from build123d import *

# Parameters (mm, degrees)
SKETCH_1_R               = 6
EXTRUDE_1015_DEPTH       = 100
SKETCH_2_R               = 6.5
EXTRUDE_2_DEPTH          = 15
SKETCH_3_R               = 6
EXTRUDE_3_DEPTH          = 11
SKETCH_4_R               = 5.5
CUT_EXTRUDE_1_DEPTH      = 2
SKETCH_5_R               = 3.5
SKETCH_5_R_2             = 0.75
EXTRUDE_1402_DEPTH       = 2
SKETCH_6_W               = 1.5
SKETCH_6_H               = 0.8
EXTRUDE_1605_DEPTH       = 1
PATTERN_CIRCULAR_1_COUNT = 8


with BuildPart() as part:
    # Эскиз1 → Extrude 1015 (new body)
    with BuildSketch(Plane(origin=(0, 0, 0), x_dir=(1, 0, 0), z_dir=(0, 1, 0))):
        with Locations(Location((0, 0, 0), (0, 0, 270))):
            Circle(SKETCH_1_R)
    extrude(amount=EXTRUDE_1015_DEPTH)

    # Эскиз2 → Бобышка-Вытянуть2 (add)
    with BuildSketch(Plane(origin=(0, 100, 0), x_dir=(1, 0, 0), z_dir=(0, 1, 0))):
        with Locations(Location((0, 0, 0), (0, 0, 270))):
            Circle(SKETCH_2_R)
    extrude(amount=EXTRUDE_2_DEPTH)

    # Эскиз3 → Бобышка-Вытянуть3 (add)
    with BuildSketch(Plane(origin=(0, 115, 0), x_dir=(1, 0, 0), z_dir=(0, 1, 0))):
        with Locations(Location((0, 0, 0), (0, 0, 270))):
            Circle(SKETCH_3_R)
    extrude(amount=EXTRUDE_3_DEPTH)

    # Эскиз4 → Вырез-Вытянуть1 (cut)
    with BuildSketch(Plane.XZ):
        with Locations(Location((0, 0, 0), (0, 0, 270))):
            Circle(SKETCH_4_R)
    extrude(amount=-CUT_EXTRUDE_1_DEPTH, mode=Mode.SUBTRACT)

    # Эскиз5 → Extrude 1402 (add)
    with BuildSketch(Plane.XZ.offset(-2)):
        with Locations(Location((0, 0, 0), (0, 0, 270))):
            Circle(SKETCH_5_R)
        with Locations(Location((0, 0, 0), (0, 0, 270))):
            Circle(SKETCH_5_R_2, mode=Mode.SUBTRACT)
    extrude(amount=EXTRUDE_1402_DEPTH)

    # Эскиз6 → Extrude 1605 (add)
    with BuildSketch(Plane.XZ.offset(-2)):
        with Locations((0, 4.5)):
            Rectangle(SKETCH_6_W, SKETCH_6_H)
    extrude_1605 = extrude(amount=EXTRUDE_1605_DEPTH)

    # Круговой массив1: Extrude 1605 ×8 about axis
    pattern_circular_1_axis = Axis((0, 0, 0), (0, 1, 0))
    for i in range(1, PATTERN_CIRCULAR_1_COUNT):
        add(extrude_1605.rotate(pattern_circular_1_axis, i * 360 / PATTERN_CIRCULAR_1_COUNT))


solid = part.part
Build history of the part. All positions in model axes, mm. A direction names the side the tool comes from. Give positions to 0.01 mm unless a question says otherwise; leave off trailing zeros. Loops run counter-clockwise (first coordinate to the right, second up) from the corner with the lowest first, then second, coordinate; pieces in that order, holes last. Notation, with made-up numbers: (55, 39.5) -> (64, 39.5) arc R26 ccw to (64, 74.5) -> close; hole circle Ø11 at (68, 46.25). An arc over 180 degrees is marked (long way). Answer in a Markdown table with one row per item.
Item 1: Tool access for faces 1 (the flat face through (3.7, 2, 0.1)), 2 (the cylindrical face through (1.802, 120.423, 5.723)), 3 (the cylindrical face through (-3.955, 107.395, -5.158)): list every direction of +Z, -Z, +X, -X, +Y, -Y with a clear straight run to the whole face (end or side of a thin tool).
Findings below:
| item | result |
|---|---|
| face 1 | -Y |
| face 2 | +Y |
| face 3 | +Y, -Y |
Item 2: Flat gauge pins, fed straight in: P1, Ø0.8, axis at y = 1.5, z = 0, coming from the -X side; P2, Ø1.1, axis at x = 0, y = 1.5, coming from the +Z side; P3, Ø3, axis at x = -2.5, y = 13.5, coming from the -Z side; P4, Ø6.5, axis at x = 0, z = 0, coming from the -Y side. Where does each tip first touch, or does it go through?
Findings below:
| item | result |
|---|---|
| P1 | stops at x = -6 |
| P2 | stops at z = 6 |
| P3 | stops at z = -5.92 |
| P4 | stops at y = 0 |
Item 3: Mould opens along X. For faces 4 (the cylindrical face through (1.802, 49.3, 5.723)), 5 (the cylindrical face through (-3.417, 1.014, 0.759)), 6 (the flat face through (1, 0, 0)) say: pulls with the +X half, pulls with the -X half, needs draft (parallel to the pull), parting line crosses it, or undercut.
Findings below:
| item | result |
|---|---|
| face 4 | parting line crosses it |
| face 5 | undercut |
| face 6 | needs draft |
Item 4: Slice it at A-A on y = 106. Write the cut outline in (x, z), plus the area to 3 significant figures.
Findings below:
| item | result |
|---|---|
| outline | circle Ø13 at (0, 0) |
| area | 133 mm² |
Item 5: Slice it at B-B on y = 35. Write the cut outline in (x, z).
Findings below:
| item | result |
|---|---|
| outline | circle Ø12 at (0, 0) |
Item 6: Probe line 1 along X through (y, z) = (0.8, 0); line 2 along X through (y, z) = (1.05, 0); line 3 along Y through (x, z) = (-3.25, 2). List the from-to ranges inside material, lowest first. Write a range as [from, to].
Findings below:
| item | result |
|---|---|
| line 1 | x = [-6, -5.5], [-3.5, -0.75], [0.75, 3.5], [5.5, 6] |
| line 2 | x = [-6, -5.5], [-4.9, -4.1], [-3.5, -0.75], [0.75, 3.5], [4.1, 4.9], [5.5, 6] |
| line 3 | y = [2, 126] |
